Model file for the job. Use its own axes, mm. A direction names the side the tool comes from. Round coordinates to 2 decimals unless told otherwise and drop trailing zeros. Order: outer loops, then holes, each group sorted by start corner. A loop starts at its lowest first (then second) coordinate and runs counter-clockwise, first axis right, second up. Notation, with made-up numbers: (53.25, 37) -> (57.25, 37) arc R32 cw to (57.25, 71) -> close; hole circle Ø6 at (53, 74.5). An arc over 180 degrees is marked (long way). Use CSV: the item, a comma, the result in double quotes.
```python
from build123d import *

# Parameters (mm, degrees)
F1_DEPTH = 95
F3_DEPTH = 10.001
F4_W     = 57
F4_H     = 24
F6_DEPTH = 180
F7_W     = 57
F7_H     = 24
F8_DEPTH = 56.001
F9_DEPTH = 179


# Not quite as in the source:
# - an extrude ends at something that could not be found from the text; its depth is read off the source's solid
# - a feature of the source that left no trace in its solid (it failed there, or was rolled back) is left out
# - a feature names something its author has since deleted; it is built from what else it names


with BuildPart() as f1:
    # F0 (on Right) → F1 (new body)
    with BuildSketch(Plane.YZ):
        Polygon((0, 56), (-10, 56), (-10, 28), (-60, 13), (-60, 0), (0, 0), align=None)
    extrude(amount=F1_DEPTH)

    # F2 (on face) → F3 (cut, through all)
    with BuildSketch(Plane.XZ.offset(10)):
        Polygon((95, 56), (57, 56), (95, 28), align=None)
    extrude(amount=-F3_DEPTH, mode=Mode.SUBTRACT)

    # F4 (on face) → F6 (cut, through all)
    with BuildSketch(Plane(origin=(0, 0, 0), x_dir=(1, 0, 0), z_dir=(0, 0, -1))):
        with Locations((47.5, 48)):
            Rectangle(F4_W, F4_H)
    extrude(amount=F6_DEPTH, mode=Mode.SUBTRACT)

    # F7 (on face) → F8 (cut, through all)
    with BuildSketch(Plane(origin=(0, 0, 0), x_dir=(1, 0, 0), z_dir=(0, 0, -1))):
        with Locations((47.5, 48)):
            Rectangle(F7_W, F7_H)
    extrude(amount=-F8_DEPTH, mode=Mode.SUBTRACT)

    # F4 (on face) → F9 (cut, through all)
    with BuildSketch(Plane(origin=(0, 0, 0), x_dir=(1, 0, 0), z_dir=(0, 0, -1))):
        with Locations((47.5, 48)):
            Rectangle(F4_W, F4_H)
    extrude(amount=F9_DEPTH, mode=Mode.SUBTRACT)


solid = f1.part
```
Q1. Cut at D-D (y = -8.5). Give the cut face in (x, z), plus the area to 3 significant figures.
From the geometry:
outline,"(0, 0) -> (95, 0) -> (95, 28) -> (57, 56) -> (0, 56) -> close"
area,"4,790 mm²"
Q2. Cut at A-A (y = -50). Give the cut face in (x, z), plus the area to 3 significant figures.
From the geometry:
outline,"(0, 0) -> (19, 0) -> (19, 16) -> (0, 16) -> close; (76, 0) -> (95, 0) -> (95, 16) -> (76, 16) -> close"
area,"608 mm²"
Q3. Which spindle directions (+Z, -Z, +X, -X, +Y, -Y) get a long thin tool onto all of the face, cutting with end or side? Do faces 1 (the flat face through (28, -5, 56)), 2 (the flat face through (36, -10, 42)), 3 (the flat face through (76, -48, 8)). Say none if no direction does.
From the geometry:
face 1,"+Z, +X, -X, +Y, -Y"
face 2,"+Z, +X, -X, -Y"
face 3,"+Z, -Z, -Y"
Q4. Probe line 1 along Y through (x, z) = (38, 39.5); line 2 along Y through (x, z) = (20, 3); line 3 along Z through (x, y) = (13.5, -36). List the from-to ranges inside material, lowest first.
From the geometry:
line 1,"y = -10 to 0"
line 2,"y = -36 to 0"
line 3,"z = 0 to 20.2"
Q5. Cut at B-B (z = 19). Give the cut face in (x, y), plus the area to 3 significant figures.
From the geometry:
outline,"(0, -40) -> (19, -40) -> (19, -36) -> (76, -36) -> (76, -40) -> (95, -40) -> (95, 0) -> (0, 0) -> close"
area,"3,570 mm²"
Q6. Cut at C-C (x = 37). Give the cut face in (y, z), plus the area to 3 significant figures.
From the geometry:
outline,"(-36, 0) -> (0, 0) -> (0, 56) -> (-10, 56) -> (-10, 28) -> (-36, 20.2) -> close"
area,"1,190 mm²"
Q7. Pin check, flat tips, straight feed: pin 1 (22 mm diameter, centred on x = 43, z = 13, fed in from -Y); pin 2 (22.5 mm diameter, centred on x = 29.5, z = 46.5, fed in from -Y). Stop position of each tip, or through.
From the geometry:
pin 1,"stops at y = -36"
pin 2,"stops at y = -10"
